Design review of the part built by this model. Coordinates are the model's own, in mm. A direction names the side the tool comes from. Coordinates: 2 decimals unless noted, no trailing zeros. Loops run counter-clockwise (first coordinate to the right, second up) from the corner with the lowest first, then second, coordinate; pieces in that order, holes last. Notation, with made-up numbers: M 27.5,-12.75 L 37.5,-12.75 A10 cw 37.5,3.25 Z; hole C -29,16.25 d1. An arc over 180 degrees is marked long. Put each result on its own line as item: value. Start each with the question number.
(1) Clearance check with a flat-ended pin moving along its axis: pin 1 (3 mm diameter, centred on x = 37.5, z = 0, fed in from +Y). State where the tip first meets the part, or that it passes through.
(2) The part is to be moulded in two halves that separate along X. For faces 1 (the flat face through (-3.448, 1.405, -2.028)), 2 (the flat face through (-50, 1, 0)), 3 (the flat face through (-1, 0, 5)), say which applies: +X half, -X half, draft (parallel to the pull), parting line (faces both ways), or undercut.
(3) Take a section at A-A, the plane x = 37.5. Give the boundary of the cut face in (y, z).
(4) Take a section at B-B, the plane z = -1.5. Give the boundary of the cut face in (x, y), then the cut area to 3 significant figures.
(5) For faces 4 (the flat face through (-3.48, 1.41, 1.97)), 5 (the flat face through (-1, 2.85, 5)), list the 3-axis set-ups (+Z, -Z, +X, -X, +Y, -Y) from which the entire face can be reached by the end or side of a thin tool; tool diameter is ignored.
(6) For probe 1 along X at (y, z) = (2.65, 0); probe 2 along X at (y, z) = (2.3, 1.5); probe 3 along X at (y, z) = (2.05, 3.5), list the stretches that pass through material, from the lowest coordinate up. Write a range as [from, to].
```python
from build123d import *

# Parameters (mm, degrees)
SKETCH1_W           = 100
SKETCH1_H           = 11.7
BOSS_EXTRUDE1_DEPTH = 2.85
CUT_EXTRUDE1_DEPTH  = 51.421671928
SKETCH3_R           = 2.4
CUT_EXTRUDE2_DEPTH  = 51.421671928


with BuildPart() as part:
    # Sketch1 → Boss-Extrude1 (new body)
    with BuildSketch(Plane(origin=(0, 0, 0), x_dir=(1, 0, 0), z_dir=(0, 1, 0))):
        Rectangle(SKETCH1_W, SKETCH1_H)
    extrude(amount=BOSS_EXTRUDE1_DEPTH)

    # Sketch2 → Cut-Extrude1 (cut, through all)
    with BuildSketch(Plane.XZ):
        Polygon((-2.309401077, 4), (2.309401077, 4), (4.618802154, 0), (2.309401077, -4), (-2.309401077, -4), (-4.618802154, 0), align=None)
    extrude(amount=-CUT_EXTRUDE1_DEPTH, mode=Mode.SUBTRACT)

    # Sketch3 → Cut-Extrude2 (cut, through all)
    with BuildSketch(Plane(origin=(0, 2.85, 0), x_dir=(1, 0, 0), z_dir=(0, 1, 0))):
        with Locations(Location((-37.5, 0, 0), (0, 0, 270))):
            Circle(SKETCH3_R)
        with Locations(Location((37.5, 0, 0), (0, 0, 270))):
            Circle(SKETCH3_R)
    extrude(amount=-CUT_EXTRUDE2_DEPTH, mode=Mode.SUBTRACT)


solid = part.part
```
Computed values:
1. pin 1: passes through
2. face 1: undercut
2. face 2: -X half
2. face 3: draft
3. outline: M 0,-5.85 L 2.85,-5.85 L 2.85,-2.4 L 0,-2.4 Z; M 0,2.4 L 2.85,2.4 L 2.85,5.85 L 0,5.85 Z
4. outline: M -50,0 L -39.37,0 L -39.37,2.85 L -50,2.85 Z; M -35.63,0 L -3.75,0 L -3.75,2.85 L -35.63,2.85 Z; M 3.75,0 L 35.63,0 L 35.63,2.85 L 3.75,2.85 Z; M 39.37,0 L 50,0 L 50,2.85 L 39.37,2.85 Z
4. area: 242 mm^2
5. face 4: +Y, -Y
5. face 5: +Z, -Z, +X, -X, +Y
6. probe 1: x = [-50, -39.9], [-35.1, -4.62], [4.62, 35.1], [39.9, 50]
6. probe 2: x = [-50, -39.37], [-35.63, -3.75], [3.75, 35.63], [39.37, 50]
6. probe 3: x = [-50, -2.6], [2.6, 50]
